Can you work these out from the drawing? Everything is in mm from the part's minimum corner. A direction names the side the tool comes from. Coordinates: 2 decimals unless noted, no trailing zeros. Loops run counter-clockwise (first coordinate to the right, second up) from the corner with the lowest first, then second, coordinate; pieces in that order, holes last. Notation, with made-up numbers: (30.5, 27) - (77.5, 27) arc R24 ccw to (77.5, 56) - close; hole circle Ø1 at (68, -13). An arc over 180 degrees is marked (long way). Use CSV: the item, a comma, the result in double quotes.
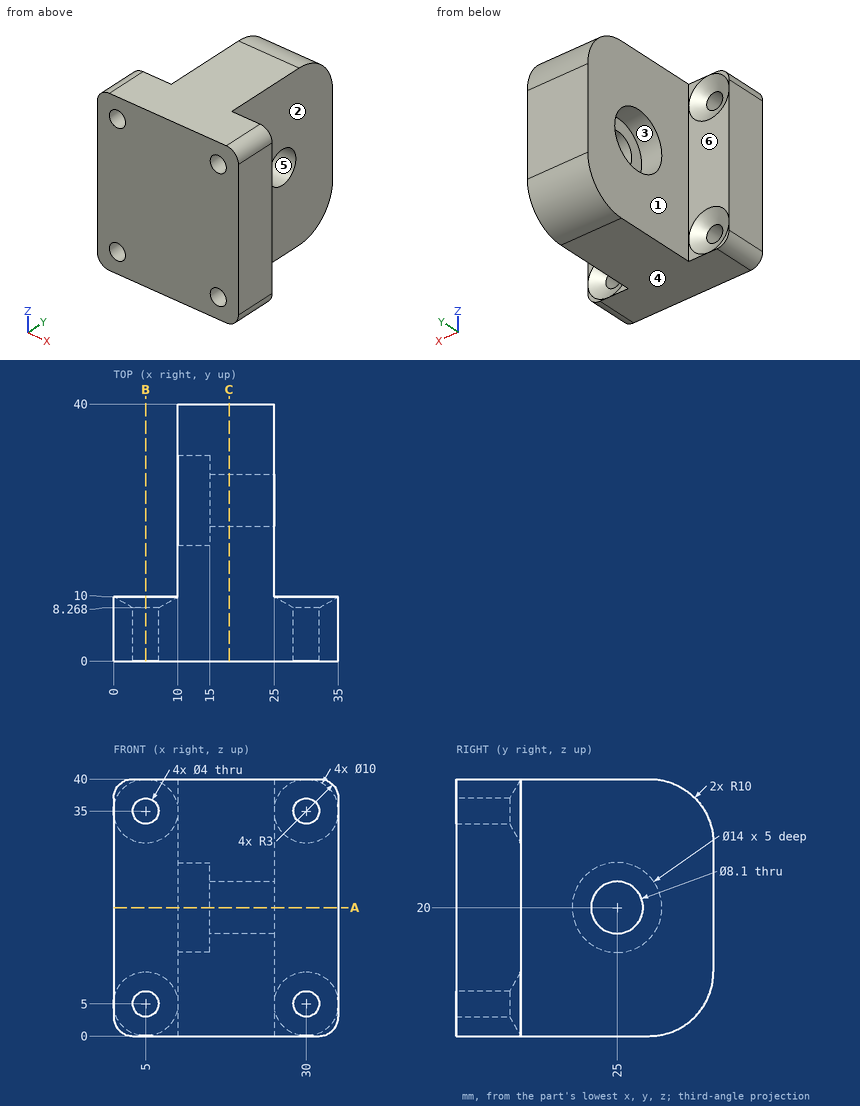
(1) Suppose I cut it at C-C (x = 18). Write out the boundary of the cut face in (y, z), plus the area to 3 significant figures.
Computed:
outline,"(0, 0) - (30, 0) arc R10 ccw to (40, 10) - (40, 30) arc R10 ccw to (30, 40) - (0, 40) - close; hole circle Ø8.1 at (25, 20)"
area,"1,510 mm²"
(2) Thinking about a two-plate mould opening in Y: for the marked faces 4, 5 and 6, which applies, +Y half, -Y half, draft (parallel to the pull), parting line (faces both ways), or undercut?
Computed:
face 4,"draft"
face 5,"undercut"
face 6,"+Y half"
(3) Suppose I cut it at B-B (x = 5). State how many separate pieces and enclosed holes the cut face has, plus the area to 3 significant figures.
Computed:
separate pieces,"3"
enclosed holes,"0"
area,"310 mm²"
(4) Which directions (+Z, -Z, +X, -X, +Y, -Y) give clear straight access to the entire face, cutting with the end or side of a thin tool? Please do the marked faces 1, 2 and 3.
Computed:
face 1,"+Z, -Z, -X, +Y"
face 2,"+Z, -Z, +X, +Y"
face 3,"-X"
(5) Will these pins go through, and if not, where does the flat tip stop? pin 1 (6 mm diameter, centred on x = 6, y = 16.5, fed in from +Z); pin 2 (3 mm diameter, centred on x = 7.5, z = 22, fed in from +Y); pin 3 (10 mm diameter, centred on y = 24.5, z = 13, fed in from +X); pin 4 (6.5 mm diameter, centred on x = 5, z = 5, fed in from +Y).
Computed:
pin 1,"passes through"
pin 2,"stops at y = 10"
pin 3,"stops at x = 25"
pin 4,"stops at y = 8.99"
(6) Please list where these lines run through material, in increasing order: line 1 (X direction, y = 4.5, z = 35); line 2 (Y direction, x = 12.65, z = 20); line 3 (Z direction, x = 4, y = 9).
Computed:
line 1,"x = 0 to 3, 7 to 28, 32 to 35"
line 2,"y = 0 to 18, 32 to 40"
line 3,"z = 0 to 1.89, 8.11 to 31.89, 38.11 to 40"
(7) Suppose I cut it at A-A (z = 20). Write out the boundary of the cut face in (x, y), plus the area to 3 significant figures.
Computed:
outline,"(0, 0) - (35, 0) - (35, 10) - (25, 10) - (25, 20.95) - (15, 20.95) - (15, 18) - (10, 18) - (10, 10) - (0, 10) - close; (10, 32) - (15, 32) - (15, 29.05) - (25, 29.05) - (25, 40) - (10, 40) - close"
area,"649 mm²"
